For this review, take the finished solid that the model builds, in its own axes (mm). A direction names the side the tool comes from. Coordinates: 2 decimals unless noted, no trailing zeros. Order: outer loops, then holes, each group sorted by start corner. A loop starts at its lowest first (then second) coordinate and runs counter-clockwise, first axis right, second up. Notation, with made-up numbers: (-30, 60.25) -> (27, 60.25) arc R15 ccw to (27, 69.25) -> close; hole circle Ø6 at (4.25, -40). An arc over 180 degrees is marked (long way). Write item = value, one per line. Start each with the question number.
1) Machinability: for faces 1 (the face through (-5.19, -7.09, -0.93)), 2 (the face through (0.065, -6.324, 4.032)), which of the approach directions +Z, -Z, +X, -X, +Y, -Y give a long, thin tool a straight path to every point of the face, cutting with its end or side? Answer none if there is none.
2) Wall thickness on probe 1 along Y at (x, z) = (1, 0); probe 2 along X at (y, z) = (6.75, -3); probe 3 along Z at (x, y) = (-7, 0.5): over which ranges is each line inside the solid? List them lowest first. Write a range as [from, to].
3) Consider section B-B on x = -6.75. Give the boundary of the cut face in (y, z).
4) Insertion check: pin 1 Ø3 at (x, y) = (-3.5, 3.5) entering from -Z; pin 2 Ø2 at (x, z) = (-1, 3.5) entering from -Y. Each pin has a flat end and moves straight along its axis. Give the tip position at first contact, or say it passes through.
5) Consider section A-A on y = 0. Give the boundary of the cut face in (x, z).
6) Draft analysis for pull direction X (two halves, no side actions). For faces 3 (the face through (6.941, -6.324, 4.032)), 4 (the face through (-8.5, 3, -3)), 5 (the face through (5.21, -7.09, -0.93)), state which applies: +X half, -X half, draft (parallel to the pull), parting line (faces both ways), or undercut.
from build123d import *

# Parameters (mm, degrees)
SKETCH_1_W = 17
SKETCH_1_H = 3.5
SKETCH_2_W = 1.1
SKETCH_2_H = 0.35
FILLET_1_R = 0.4


with BuildPart() as part:
    # 草图1 → 旋转1 (revolve)
    with BuildSketch(Plane.XY, mode=Mode.PRIVATE) as revolve_1_sk:
        with Locations((0, 5.75)):
            Rectangle(SKETCH_1_W, SKETCH_1_H)
    revolve(revolve_1_sk.sketch.rotate(Axis((0, 0, 0), (1, 0, 0)), 90), axis=Axis((0, 0, 0), (1, 0, 0)))

    # 草图2 → 切除-旋转1 (revolve, cut)
    with BuildSketch(Plane.XY, mode=Mode.PRIVATE) as cut_revolve_1_sk:
        with Locations((-5.2, 7.325)):
            Rectangle(SKETCH_2_W, SKETCH_2_H)
        with Locations((5.2, 7.325)):
            Rectangle(SKETCH_2_W, SKETCH_2_H)
    revolve(cut_revolve_1_sk.sketch.rotate(Axis((0, 0, 0), (1, 0, 0)), 90), axis=Axis((0, 0, 0), (1, 0, 0)), mode=Mode.SUBTRACT)

    # 圆角1
    fillet_1_edges = [part.edges().sort_by_distance(p)[0] for p in [
        (-8.5, 0, -7.5),
        (8.5, 0, -7.5),
    ]]
    fillet(fillet_1_edges, radius=FILLET_1_R)


solid = part.part
Answer sheet:
q1.face_1 = none
q1.face_2 = +X, -X
q2.probe_1 = [-7.5, -4], [4, 7.5]
q2.probe_2 = [-8.38, -5.75], [-4.65, 4.65], [5.75, 8.38]
q2.probe_3 = [-7.48, -3.97], [3.97, 7.48]
q3.outline = circle Ø15 at (0, 0); hole circle Ø8 at (0, 0)
q4.pin_1 = -7.23
q4.pin_2 = -7.07
q5.outline = (-8.5, -7.1) arc R0.4 ccw to (-8.1, -7.5) -> (-5.75, -7.5) -> (-5.75, -7.15) -> (-4.65, -7.15) -> (-4.65, -7.5) -> (4.65, -7.5) -> (4.65, -7.15) -> (5.75, -7.15) -> (5.75, -7.5) -> (8.1, -7.5) arc R0.4 ccw to (8.5, -7.1) -> (8.5, -4) -> (-8.5, -4) -> close; (-8.5, 4) -> (8.5, 4) -> (8.5, 7.1) arc R0.4 ccw to (8.1, 7.5) -> (5.75, 7.5) -> (5.75, 7.15) -> (4.65, 7.15) -> (4.65, 7.5) -> (-4.65, 7.5) -> (-4.65, 7.15) -> (-5.75, 7.15) -> (-5.75, 7.5) -> (-8.1, 7.5) arc R0.4 ccw to (-8.5, 7.1) -> close
q6.face_3 = draft
q6.face_4 = -X half
q6.face_5 = undercut
